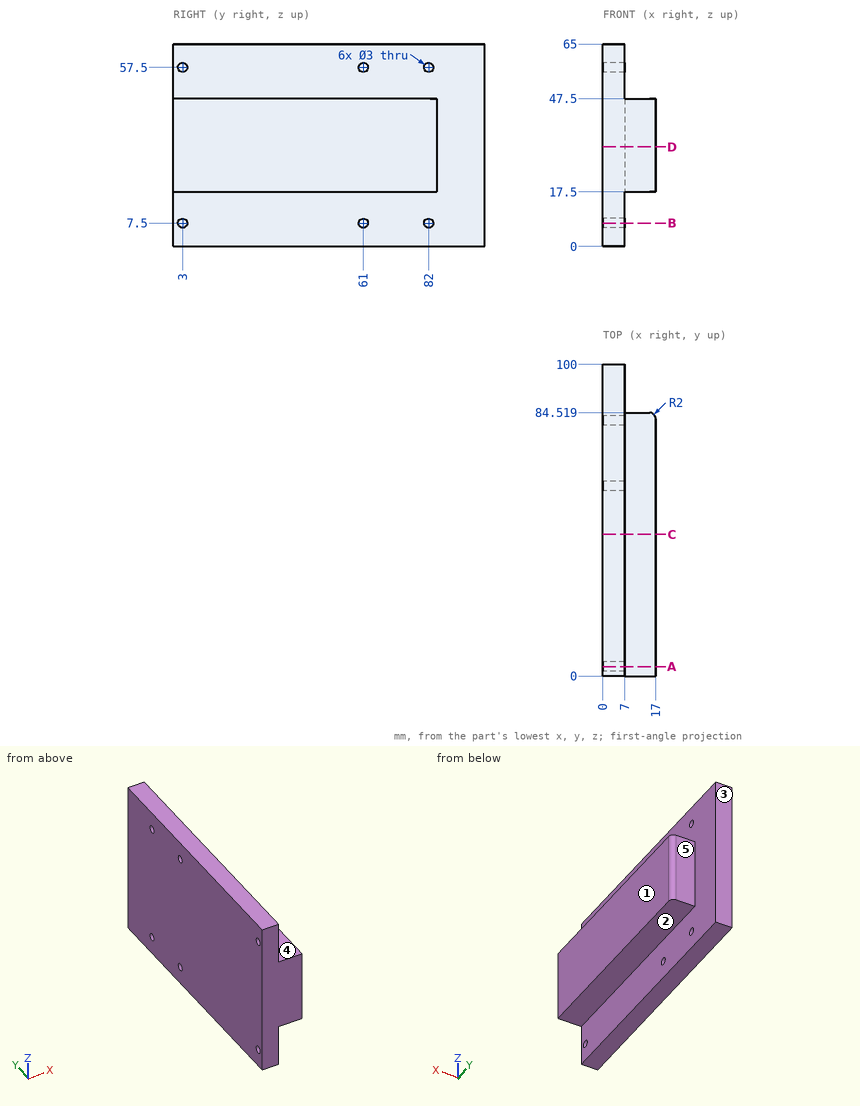
Design review of the part shown in the three views and the two pictorial views. Dimensions are in mm from the part's minimum x, y and z. A direction names the side the tool comes from. Give positions to 0.01 mm unless a question says otherwise; leave off trailing zeros. Loops run counter-clockwise (first coordinate to the right, second up) from the corner with the lowest first, then second, coordinate; pieces in that order, holes last. Notation, with made-up numbers: (59.5, 48.5) -> (106.5, 48.5) arc R35 ccw to (106.5, 84.5) -> close; hole circle Ø3 at (37.25, 42). An arc over 180 degrees is marked (long way). Put each result on its own line as item: value. Start each with the question number.
1. Clearance check with flat-ended pins moving along their axes: P1, Ø8, axis at x = 11.5, y = 42, coming from the +Z side; P2, Ø3.5, axis at y = 3, z = 7.5, coming from the +X side; P3, Ø2.5, axis at x = 10.5, z = 27, coming from the +Y side. State where each tip first meets the part, or that it passes through.
2. We need section D-D on z = 32. State the section outline as (x, y) points, then the cut area to 3 significant figures.
3. We need section C-C on y = 45.5. State the section outline as (x, z) points, then the cut area to 3 significant figures.
4. For the marked faces 1, 2, 3, 4 and 5, list the 3-axis set-ups (+Z, -Z, +X, -X, +Y, -Y) from which the entire face can be reached by the end or side of a thin tool; tool diameter is ignored.
5. We need section B-B on z = 7.5. State the section outline as (x, y) points, then the cut area to 3 significant figures.
6. We need section A-A on y = 3. State the section outline as (x, z) points.
7. Wall thickness on probe 1 along Y at (x, z) = (2.5, 57.5); probe 2 along Z at (x, y) = (5, 61); probe 3 along X at (y, z) = (95, 40.5): over which ranges is each line inside the solid? List them lowest first.
Determined:
1. P1: z = 47.5
1. P2: x = 7
1. P3: y = 84.52
2. outline: (0, 0) -> (17, 0) -> (17, 82.52) arc R2 ccw to (15, 84.52) -> (7, 84.52) -> (7, 100) -> (0, 100) -> close
2. area: 1,540 mm^2
3. outline: (0, 0) -> (7, 0) -> (7, 17.5) -> (17, 17.5) -> (17, 47.5) -> (7, 47.5) -> (7, 65) -> (0, 65) -> close
3. area: 755 mm^2
4. face 1: +Z, -Z, +X, +Y, -Y
4. face 2: -Z, +X, +Y, -Y
4. face 3: +Z, -Z, +X, -X, +Y
4. face 4: +Z, +X, +Y, -Y
4. face 5: +Z, -Z, +X, +Y
5. outline: (0, 0) -> (7, 0) -> (7, 1.5) -> (0, 1.5) -> close; (0, 4.5) -> (7, 4.5) -> (7, 59.5) -> (0, 59.5) -> close; (0, 62.5) -> (7, 62.5) -> (7, 80.5) -> (0, 80.5) -> close; (0, 83.5) -> (7, 83.5) -> (7, 100) -> (0, 100) -> close
5. area: 637 mm^2
6. outline: (0, 0) -> (7, 0) -> (7, 6) -> (0, 6) -> close; (0, 9) -> (7, 9) -> (7, 17.5) -> (17, 17.5) -> (17, 47.5) -> (7, 47.5) -> (7, 56) -> (0, 56) -> close; (0, 59) -> (7, 59) -> (7, 65) -> (0, 65) -> close
7. probe 1: 0 to 1.5, 4.5 to 59.5, 62.5 to 80.5, 83.5 to 100
7. probe 2: 0 to 6, 9 to 56, 59 to 65
7. probe 3: 0 to 7
